Geometry check sheet. Reference: the model listing, model coordinates, mm. A direction names the side the tool comes from. Coordinates: 2 decimals unless noted, no trailing zeros. Order: outer loops, then holes, each group sorted by start corner. A loop starts at its lowest first (then second) coordinate and runs counter-clockwise, first axis right, second up. Notation, with made-up numbers: M 10.5,24.25 L 44.5,24.25 A16 cw 44.5,39.25 Z; hole C 73.25,-29 d1. An arc over 180 degrees is marked long. Use CSV: the item, a comma, the result in double quotes. Start each with the question number.
```python
from build123d import *

# Parameters (mm, degrees)
CROQUIS1_W              = 250
CROQUIS1_H              = 250
CROQUIS1_R              = 2.5
SALIENTE_EXTRUIR1_DEPTH = 4
CORTAR_EXTRUIR1_DEPTH   = 4
CROQUIS3_W              = 150
CROQUIS3_H              = 150
CROQUIS3_W_2            = 100
CROQUIS3_H_2            = 100
SALIENTE_EXTRUIR2_DEPTH = 4
CROQUIS4_R              = 1.55
CORTAR_EXTRUIR2_DEPTH   = 10
CROQUIS5_W              = 150
CROQUIS5_H              = 150
CROQUIS5_W_2            = 100
CROQUIS5_H_2            = 100
CORTAR_EXTRUIR3_DEPTH   = 10
CROQUIS6_W              = 30
CROQUIS6_H              = 50
CROQUIS6_W_2            = 50
CROQUIS6_H_2            = 30
CORTAR_EXTRUIR4_DEPTH   = 10
CROQUIS8_R              = 1.55
CORTAR_EXTRUIR5_DEPTH   = 10
CROQUIS9_R              = 2.5
CROQUIS9_R_2            = 1.55
CORTAR_EXTRUIR7_DEPTH   = 10
CORTAR_EXTRUIR8_DEPTH   = 10


with BuildPart() as part:
    # Croquis1 → Saliente-Extruir1 (new body)
    with BuildSketch(Plane(origin=(0, 0, 0), x_dir=(1, 0, 0), z_dir=(0, 1, 0))):
        with Locations((125, 125)):
            Rectangle(CROQUIS1_W, CROQUIS1_H)
        with Locations(Location((40, 210, 0), (0, 0, 270))):
            Circle(CROQUIS1_R, mode=Mode.SUBTRACT)
        with Locations(Location((210, 210, 0), (0, 0, 270))):
            Circle(CROQUIS1_R, mode=Mode.SUBTRACT)
        with Locations(Location((210, 40, 0), (0, 0, 270))):
            Circle(CROQUIS1_R, mode=Mode.SUBTRACT)
        with Locations(Location((40, 40, 0), (0, 0, 270))):
            Circle(CROQUIS1_R, mode=Mode.SUBTRACT)
    extrude(amount=SALIENTE_EXTRUIR1_DEPTH)

    # Croquis2 → Cortar-Extruir1 (cut)
    with BuildSketch(Plane(origin=(0, 4, 0), x_dir=(1, 0, 0), z_dir=(0, 1, 0))):
        Polygon((50, 50), (200, 50), (200, 200), (50, 200), (50, 150.09044268), align=None)
    extrude(amount=-CORTAR_EXTRUIR1_DEPTH, mode=Mode.SUBTRACT)

    # Croquis3 → Saliente-Extruir2 (add)
    with BuildSketch(Plane(origin=(0, 4, 0), x_dir=(1, 0, 0), z_dir=(0, 1, 0))):
        with Locations((125, 125)):
            Rectangle(CROQUIS3_W, CROQUIS3_H)
        with Locations((125, 125)):
            Rectangle(CROQUIS3_W_2, CROQUIS3_H_2, mode=Mode.SUBTRACT)
    extrude(amount=-SALIENTE_EXTRUIR2_DEPTH)

    # Croquis4 → Cortar-Extruir2 (cut)
    with BuildSketch(Plane(origin=(0, 4, 0), x_dir=(1, 0, 0), z_dir=(0, 1, 0))):
        with Locations(Location((115, 20, 0), (0, 0, 270))):
            Circle(CROQUIS4_R)
        with Locations(Location((135, 20, 0), (0, 0, 270))):
            Circle(CROQUIS4_R)
        with Locations(Location((125, 5, 0), (0, 0, 270))):
            Circle(CROQUIS4_R)
    extrude(amount=-CORTAR_EXTRUIR2_DEPTH, mode=Mode.SUBTRACT)

    # Croquis5 → Cortar-Extruir3 (cut)
    with BuildSketch(Plane(origin=(0, 4, 0), x_dir=(1, 0, 0), z_dir=(0, 1, 0))):
        with Locations((125, 125)):
            Rectangle(CROQUIS5_W, CROQUIS5_H)
        with Locations((125, 125)):
            Rectangle(CROQUIS5_W_2, CROQUIS5_H_2, mode=Mode.SUBTRACT)
    extrude(amount=-CORTAR_EXTRUIR3_DEPTH, mode=Mode.SUBTRACT)

    # Croquis6 → Cortar-Extruir4 (cut)
    with BuildSketch(Plane(origin=(0, 4, 0), x_dir=(1, 0, 0), z_dir=(0, 1, 0))):
        Polygon((170, 0), (250, 0), (250, 30), (220, 30), (170, 30), align=None)
        with Locations((235, 55)):
            Rectangle(CROQUIS6_W, CROQUIS6_H)
        Polygon((0, 80), (0, 0), (30, 0), (30, 30), (30, 80), align=None)
        with Locations((55, 15)):
            Rectangle(CROQUIS6_W_2, CROQUIS6_H_2)
        Polygon((80, 250), (0, 250), (0, 220), (30, 220), (80, 220), align=None)
        with Locations((15, 195)):
            Rectangle(CROQUIS6_W, CROQUIS6_H)
        Polygon((250, 170), (250, 250), (220, 250), (220, 220), (220, 170), align=None)
        with Locations((195, 235)):
            Rectangle(CROQUIS6_W_2, CROQUIS6_H_2)
    extrude(amount=-CORTAR_EXTRUIR4_DEPTH, mode=Mode.SUBTRACT)

    # Croquis8 → Cortar-Extruir5 (cut)
    with BuildSketch(Plane(origin=(0, 4, 0), x_dir=(1, 0, 0), z_dir=(0, 1, 0))):
        with Locations(Location((125, 5, 0), (0, 0, 270))):
            Circle(CROQUIS8_R)
        with Locations(Location((135, 20, 0), (0, 0, 270))):
            Circle(CROQUIS8_R)
        with Locations(Location((115, 20, 0), (0, 0, 270))):
            Circle(CROQUIS8_R)
        with Locations(Location((20, 135, 0), (0, 0, 270))):
            Circle(CROQUIS8_R)
        with Locations(Location((5, 125, 0), (0, 0, 270))):
            Circle(CROQUIS8_R)
        with Locations(Location((20, 115, 0), (0, 0, 270))):
            Circle(CROQUIS8_R)
        with Locations(Location((135, 230, 0), (0, 0, 270))):
            Circle(CROQUIS8_R)
        with Locations(Location((125, 245, 0), (0, 0, 270))):
            Circle(CROQUIS8_R)
        with Locations(Location((115, 230, 0), (0, 0, 270))):
            Circle(CROQUIS8_R)
        with Locations(Location((230, 115, 0), (0, 0, 270))):
            Circle(CROQUIS8_R)
        with Locations(Location((245, 125, 0), (0, 0, 270))):
            Circle(CROQUIS8_R)
        with Locations(Location((230, 135, 0), (0, 0, 270))):
            Circle(CROQUIS8_R)
    extrude(amount=-CORTAR_EXTRUIR5_DEPTH, mode=Mode.SUBTRACT)

    # Croquis9 → Cortar-Extruir7 (cut)
    # profile 1 of 2: a face of its own
    with BuildSketch(Plane(origin=(0, 4, 0), x_dir=(1, 0, 0), z_dir=(0, 1, 0))):
        Polygon((30, 30), (50, 30), (50, 34), (53, 34), (53, 46), (50, 46), (50, 50), (50, 200), (50, 204), (53, 204), (53, 216), (50, 216), (50, 220), (30, 220), (30, 170), (0, 170), (0, 80), (30, 80), align=None)
        with Locations((40, 40)):
            Circle(CROQUIS9_R, mode=Mode.SUBTRACT)
        with Locations((20, 115)):
            Circle(CROQUIS9_R_2, mode=Mode.SUBTRACT)
        with Locations((5, 125)):
            Circle(CROQUIS9_R_2, mode=Mode.SUBTRACT)
        with Locations((20, 135)):
            Circle(CROQUIS9_R_2, mode=Mode.SUBTRACT)
        with Locations((40, 210)):
            Circle(CROQUIS9_R, mode=Mode.SUBTRACT)
    # profile 2 of 2: a face of its own
    with BuildSketch(Plane(origin=(0, 4, 0), x_dir=(1, 0, 0), z_dir=(0, 1, 0))):
        Polygon((200, 0), (250, 0), (250, 250), (200, 250), (200, 216), (197, 216), (197, 204), (200, 204), (200, 46), (197, 46), (197, 34), (200, 34), align=None)
    extrude(amount=-CORTAR_EXTRUIR7_DEPTH, mode=Mode.SUBTRACT)


with BuildPart() as cortar_extruir7_piece_1:
    # of the separate pieces the step leaves, piece 1, a body of its own (cortar_extruir7_pieces)
    add(part.part.solids().sort_by_distance((80, 0, 0))[0])

    # Croquis10 → Cortar-Extruir8 (cut)
    with BuildSketch(Plane(origin=(0, 4, 0), x_dir=(1, 0, 0), z_dir=(0, 1, 0))):
        Polygon((200, 50), (50, 50), (50, 46), (53, 46), (53, 34), (50, 34), (50, 30), (80, 30), (80, 0), (170, 0), (170, 30), (200, 30), (200, 34), (197, 34), (197, 46), (200, 46), align=None)
    extrude(amount=-CORTAR_EXTRUIR8_DEPTH, mode=Mode.SUBTRACT)


with BuildPart() as cortar_extruir7_piece_2:
    # of the separate pieces the step leaves, piece 2, a body of its own (cortar_extruir7_pieces)
    add(part.part.solids().sort_by_distance((50, 0, -200))[0])


solid = cortar_extruir7_piece_2.part
```
1) Section check D-D on z = -233. Record the boundary of the cut face in (x, y), then the cut area to 3 significant figures.
2) Section check B-B on x = 115. Record the boundary of the cut face in (y, z).
3) Draft check along Z on faces 6 (the face through (124, 2, -250)), 7 (the face through (200, 2, -218)), 8 (the face through (134.06, 2.03, -231.23)). Enter one of: +Z half, -Z half, draft (parallel to the pull), parting line (faces both ways), or undercut.
4) Gauge pin test, flat ends, axial feed: P1, Ø1.5, axis at x = 52, y = 3, coming from the -Z side; P2, Ø1.9, axis at x = 125, z = -245, coming from the +Y side; P3, Ø1.2, axis at y = 3, z = -236.5, coming from the +X side; P4, Ø1.2, axis at y = 1.5, z = -210.5, coming from the +X side. Record the tip position at first contact, or that the pin passes through.
5) Material ranges on line 1 along X through (y, z) = (0.9, -230); line 2 along Z through (x, y) = (125, 2.25); line 3 along Z through (x, y) = (135, 2.45), recorded low to high.
6) Set-up check for faces 1 (the face through (51, 2, -204)), 2 (the face through (65, 2, -220)), 3 (the face through (198, 2, -204)), 4 (the face through (200, 2, -202)), 5 (the face through (170, 2, -235)): record each of +Z, -Z, +X, -X, +Y, -Y from which the full face is reachable in a straight line by a thin tool's end or side.
7) Section check C-C on y = 1.8. Record the boundary of the cut face in (x, z), then the cut area to 3 significant figures.
8) Section check A-A on z = -245. Record the boundary of the cut face in (x, y).
Results are:
1,outline,"M 80,0 L 170,0 L 170,4 L 80,4 Z"
1,area,"360 mm²"
2,outline,"M 0,-250 L 4,-250 L 4,-231.55 L 0,-231.55 Z; M 0,-228.45 L 4,-228.45 L 4,-200 L 0,-200 Z"
3,face 6,"-Z half"
3,face 7,"draft"
3,face 8,"undercut"
4,P1,"stops at z = -220"
4,P2,"passes through"
4,P3,"stops at x = 170"
4,P4,"stops at x = 197"
5,line 1,"x = 80 to 113.45, 116.55 to 133.45, 136.55 to 170"
5,line 2,"z = -250 to -246.55, -243.45 to -200"
5,line 3,"z = -250 to -231.55, -228.45 to -200"
6,face 1,"-X, +Y, -Y"
6,face 2,"-Z, -X, +Y, -Y"
6,face 3,"+X, +Y, -Y"
6,face 4,"+Z, -Z, +X, +Y, -Y"
6,face 5,"-Z, +X, +Y, -Y"
7,outline,"M 50,-220 L 80,-220 L 80,-250 L 170,-250 L 170,-220 L 200,-220 L 200,-216 L 197,-216 L 197,-204 L 200,-204 L 200,-200 L 50,-200 L 50,-204 L 53,-204 L 53,-216 L 50,-216 Z; hole C 115,-230 d3.1; hole C 125,-245 d3.1; hole C 135,-230 d3.1"
7,area,"5,610 mm²"
8,outline,"M 80,0 L 123.45,0 L 123.45,4 L 80,4 Z; M 126.55,0 L 170,0 L 170,4 L 126.55,4 Z"
